Study the drawing (mm; zero at the part's minimum x, y, z) and answer. A direction names the side the tool comes from. Round coordinates to 2 decimals unless told otherwise and drop trailing zeros. Write each loop counter-clockwise with the first axis right and the second up, starting at its lowest first coordinate (ties: lowest second). Pieces come first, ordered by that corner, then holes. Notation, with made-up numbers: (67, -13.5) -> (86, -13.5) arc R24 cw to (86, 23.5) -> close; hole circle Ø8 at (14.5, 42.5). An arc over 180 degrees is marked (long way). Write each question's results on one line, items separated by ' | '. Start each with the question number.
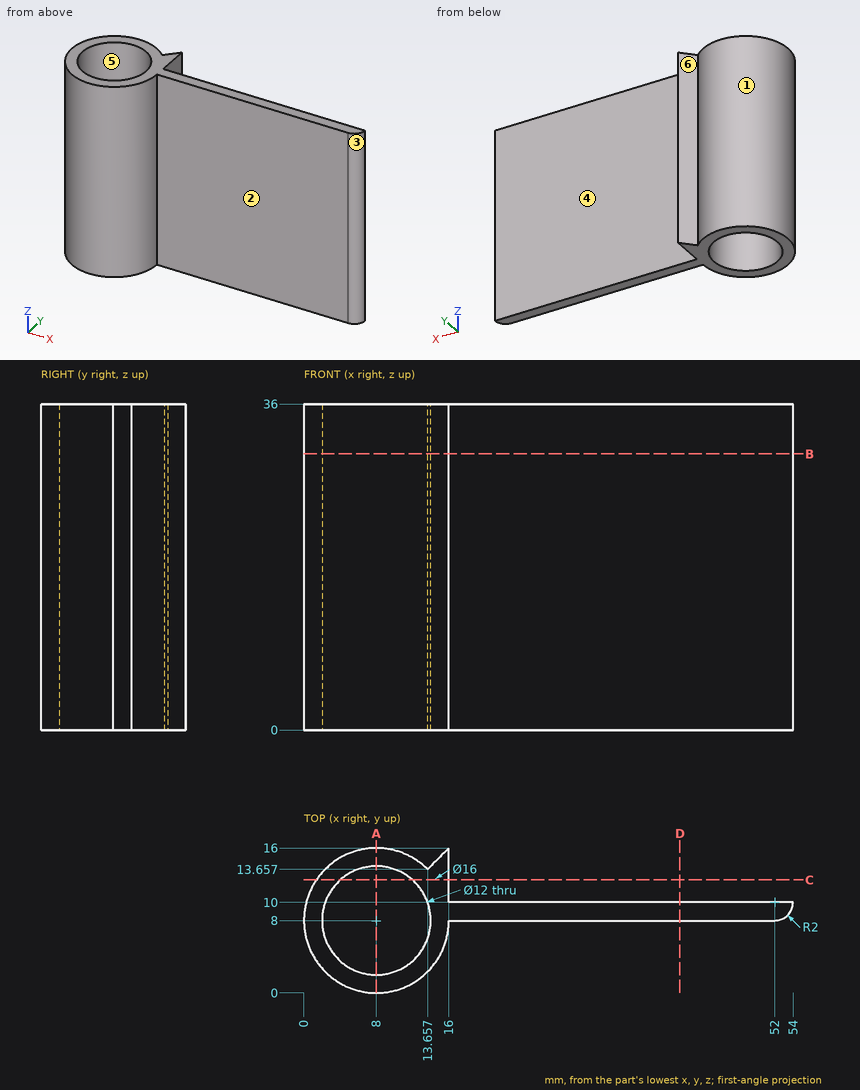
Q1. For the marked faces 1 and 2, determine the directions among +Z, -Z, +X, -X, +Y, -Y from which every point of the face is accessible in a straight line to the end or side of a thin tool.
Q2. Find the intervals of material crossed by line 1 (Y direction, x = 8, z = 9); line 2 (Y direction, x = 49, z = 22); line 3 (X direction, y = 4, z = 19.5), in increasing order.
Q3. The part is cut by section C-C, the plane y = 12.5. Write down the section's boundary in (x, z).
Q4. The part is cut by section A-A, the plane x = 8. Write down the section's boundary in (y, z).
Q5. Determine the mould class of the marked faces 3, 4, 5 and 6 for opening direction X: pulls with the +X half, pulls with the -X half, needs draft (parallel to the pull), parting line crosses it, or undercut.
Q6. The part is cut by section B-B, the plane z = 30.5. Write down the section's boundary in (x, y).
Q7. The part is cut by section D-D, the plane x = 41.5. Write down the section's boundary in (y, z), then the cut area to 3 significant figures.
Q8. Each of these flat-tipped pins is pushed along its axis until it touches: pin 1 (2 mm diameter, centred on x = 45.5, z = 16, fed in from -Y); pin 2 (5 mm diameter, centred on y = 14.5, z = 15.5, fed in from +X); pin 3 (1 mm diameter, centred on y = 2, z = 13.5, fed in from -X). Where does it stop, or does it pass through?
Answers follow:
1) face 1: +Z, -Z | face 2: +Z, -Z, +X, -Y
2) line 1: 0 to 2, 14 to 16 | line 2: 8 to 10 | line 3: 1.07 to 3.53, 12.47 to 14.93
3) outline: (1.39, 0) -> (4.03, 0) -> (4.03, 36) -> (1.39, 36) -> close; (11.97, 0) -> (16, 0) -> (16, 36) -> (11.97, 36) -> close
4) outline: (0, 0) -> (2, 0) -> (2, 36) -> (0, 36) -> close; (14, 0) -> (16, 0) -> (16, 36) -> (14, 36) -> close
5) face 3: pulls with the +X half | face 4: needs draft | face 5: undercut | face 6: undercut
6) outline: (13.66, 13.66) arc R8 ccw (long way) to (16, 8) -> (52, 8) arc R2 ccw to (54, 10) -> (16, 10) -> (16, 16) -> close; hole circle Ø12 at (8, 8)
7) outline: (8, 0) -> (10, 0) -> (10, 36) -> (8, 36) -> close | area: 72.0 mm^2
8) pin 1: y = 8 | pin 2: x = 16 | pin 3: x = 2.19
